Input: dimensioned drawing with shaded views. Units: mm. Origin: part minimum x, y, z. Coordinates: 2 decimals unless noted, no trailing zeros. Order: outer loops, then holes, each group sorted by start corner. A loop starts at its lowest first (then second) coordinate and runs counter-clockwise, first axis right, second up. Notation, with made-up numbers: M 68.25,70.5 L 116.25,70.5 A21 cw 116.25,95.5 Z; hole C 66.25,82 d4. An arc over 180 degrees is marked long. Write item = value, one per line.
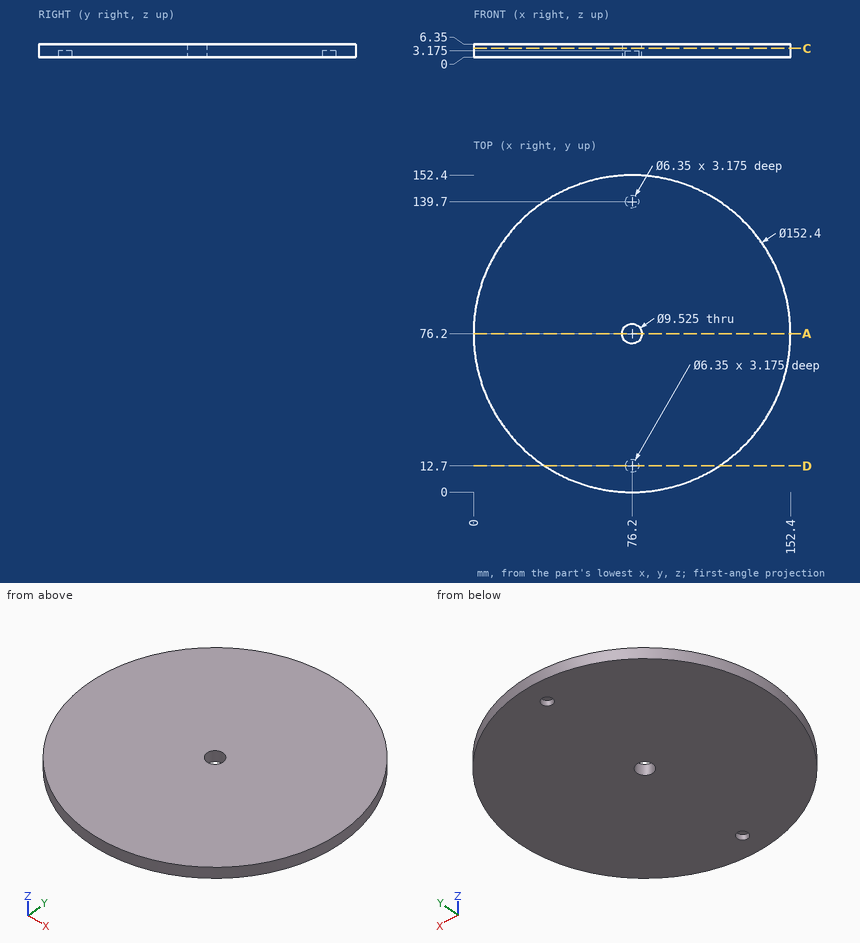
1) Pin query (flat end, axial travel): pin 1 (7 mm diameter, centred on x = 75.5, y = 12, fed in from -Z); pin 2 (1 mm diameter, centred on x = 64, z = 5, fed in from +Y); pin 3 (3 mm diameter, centred on x = 83.5, z = 4.5, fed in from -Y); pin 4 (3 mm diameter, centred on x = 65, z = 3.5, fed in from +Y). Return the tip coordinate at first contact, or that it passes through.
Numbers:
pin_1 = 0
pin_2 = 151.5
pin_3 = 0.22
pin_4 = 151.78
2) Section C-C, the plane z = 4.25. Return loops of the section in (x, y) (1 decimal), and give its area (3 significant figures).
Numbers:
outline = C 76.2,76.2 d152.4; hole C 76.2,76.2 d9.5
area = 18,200 mm²
3) Line query: L1, parallel to Y at x = 76.2, z = 2 (1 decimal); L2, parallel to Y at x = 75, z = 1.75; L3, parallel to X at y = 79, z = 1. Output: solid intervals per line, ascending.
Numbers:
L1 = 0 to 9.5, 15.9 to 71.4, 81 to 136.5, 142.9 to 152.4
L2 = 0.01 to 9.76, 15.64 to 71.59, 80.81 to 136.76, 142.64 to 152.39
L3 = 0.05 to 72.35, 80.05 to 152.35
4) Section A-A, the plane y = 76.2. Return loops of the section in (x, z).
Numbers:
outline = M 0,0 L 71.44,0 L 71.44,6.35 L 0,6.35 Z; M 80.96,0 L 152.4,0 L 152.4,6.35 L 80.96,6.35 Z
5) Section D-D, the plane y = 12.7. Return loops of the section in (x, z) (3 decimals).
Numbers:
outline = M 34.079,0 L 73.025,0 L 73.025,3.175 L 79.375,3.175 L 79.375,0 L 118.321,0 L 118.321,6.35 L 34.079,6.35 Z
